Can you work these out from the model? Positions are in its coordinate system, mm. A direction names the side the tool comes from. Round coordinates to 2 decimals unless told otherwise and drop trailing zeros. Loops run counter-clockwise (first coordinate to the right, second up) from the corner with the lowest first, then second, coordinate; pieces in that order, holes last. Notation, with made-up numbers: (44.25, -29.5) -> (95.25, -29.5) arc R33 ccw to (95.25, 6.5) -> close; hole circle Ø3 at (74, 41). An arc over 180 degrees is marked (long way). Answer as a JSON object with one key per item and string values.
```python
from build123d import *

# Parameters (mm, degrees)
F0_W      = 114.3
F0_H      = 69.85
F1_DEPTH  = 50.8
F3_DEPTH  = 76.2
F4_DEPTH  = 19.05
F6_DEPTH  = 12.7
F8_DEPTH  = 76.2
F10_DEPTH = 38.1
F12_DEPTH = 76.2
F14_DEPTH = 12.7
F15_R     = 3.175
F16_DEPTH = 76.2


with BuildPart() as f1:
    # F0 (on Front) → F1 (new body)
    with BuildSketch(Plane.XZ):
        with Locations((57.15, 34.925)):
            Rectangle(F0_W, F0_H)
    extrude(amount=-F1_DEPTH)

    # F2 (on face) → F3 (cut)
    with BuildSketch(Plane.XZ):
        Polygon((0, 0), (63.5, 0), (0, 31.75), align=None)
    extrude(amount=-F3_DEPTH, mode=Mode.SUBTRACT)

    # F2 (on face) → F4 (cut)
    with BuildSketch(Plane.XZ):
        Polygon((38.1, 69.85), (114.3, 50.8), (114.3, 69.85), align=None)
    extrude(amount=-F4_DEPTH, mode=Mode.SUBTRACT)

    # F5 (on face) → F6 (cut)
    with BuildSketch(Plane(origin=(0, 50.8, 0), x_dir=(-1, 0, 0), z_dir=(0, 1, 0))):
        Polygon((-114.3, 50.8), (-38.1, 69.85), (-114.3, 69.85), align=None)
    extrude(amount=-F6_DEPTH, mode=Mode.SUBTRACT)

    # F7 (on face) → F8 (cut)
    with BuildSketch(Plane.XZ.offset(-19.05)):
        Polygon((101.6, 53.975), (101.6, 69.85), (38.1, 69.85), align=None)
    extrude(amount=-F8_DEPTH, mode=Mode.SUBTRACT)

    # F9 (on face) → F10 (join)
    with BuildSketch(Plane.YZ.offset(114.3)):
        Polygon((38.1, 69.85), (19.05, 69.85), (19.05, 50.8), (19.05, 0), (50.8, 0), (50.8, 50.8), (38.1, 50.8), align=None)
    extrude(amount=F10_DEPTH)

    # F11 (on face) → F12 (cut)
    with BuildSketch(Plane.XZ.offset(-19.05)):
        Polygon((139.7, 69.85), (139.7, 31.75), (152.4, 25.4), (152.4, 69.85), align=None)
    extrude(amount=-F12_DEPTH, mode=Mode.SUBTRACT)

    # F13 (on face) → F14 (cut)
    with BuildSketch(Plane(origin=(0, 50.8, 0), x_dir=(-1, 0, 0), z_dir=(0, 1, 0))):
        Polygon((-139.7, 31.75), (-114.3, 50.8), (-139.7, 50.8), align=None)
    extrude(amount=-F14_DEPTH, mode=Mode.SUBTRACT)

    # F15 (on face) → F16 (cut)
    with BuildSketch(Plane.XY.offset(69.85)):
        with Locations((111.125, 28.575)):
            Circle(F15_R)
        with Locations((130.175, 28.575)):
            Circle(F15_R)
    extrude(amount=-F16_DEPTH, mode=Mode.SUBTRACT)


solid = f1.part
```
Q1. I'm going to push flat-ended pins straight in: pin 1 (9.5 mm diameter, centred on y = 31, z = 43, fed in from +X); pin 2 (9.5 mm diameter, centred on y = 13, z = 25.5, fed in from +X); pin 3 (1 mm diameter, centred on y = 40, z = 50, fed in from +X). Where does each tip first touch, or does it pass through?
Determined:
{"pin 1": "x = 139.7", "pin 2": "x = 114.3", "pin 3": "x = 116.03"}
Q2. We'd pull the mould along X, two halves only. Please class faces 6 (the flat face through (139.7, 28, 51)), 7 (the flat face through (125, 38.1, 55)), 8 (the cylindrical face through (133.11, 27.36, 35.41)): pulls with the +X half, pulls with the -X half, needs draft (parallel to the pull), parting line crosses it, or undercut.
Determined:
{"face 6": "pulls with the +X half", "face 7": "needs draft", "face 8": "undercut"}
Q3. I want a section at B-B, the plane x = 111. Write out the boundary of the cut face in (y, z) (3 decimals), then the cut area to 3 significant figures.
Determined:
{"outline": "(0, 0) -> (25.402, 0) -> (25.402, 69.85) -> (19.05, 69.85) -> (19.05, 51.625) -> (0, 51.625) -> close; (31.748, 0) -> (50.8, 0) -> (50.8, 51.625) -> (38.1, 51.625) -> (38.1, 69.85) -> (31.748, 69.85) -> close", "area": "2,530 mm²"}
Q4. On a 3-axis mill with a long thin cutter (end or side, diameter ignored), from which of +Z, -Z, +X, -X, +Y, -Y can I reach the whole of each face in a straight line? I mean faces 1 (the flat face through (127.18, 44.54, 41.14)), 2 (the flat face through (152.4, 35, 13)), 3 (the cylindrical face through (114.06, 27.36, 35.41)), 4 (the flat face through (101.6, 28, 62)), 5 (the flat face through (114.3, 9, 25)). Say none if no direction works.
Determined:
{"face 1": "+Z, +X, +Y", "face 2": "+Z, -Z, +X, +Y, -Y", "face 3": "+Z, -Z", "face 4": "+Z, +Y, -Y", "face 5": "+Z, -Z, +X, -Y"}
Q5. If I drill on L1, parallel to X at y = 26.5, z = 41.5; L2, parallel to X at y = 31, z = 45; L3, parallel to Y at x = 134.5, z = 32.5, over which ranges is the centre line in solid material (lowest first)? Write a range as [from, to].
Determined:
{"L1": "[0, 108.72], [113.53, 127.77], [132.58, 139.7]", "L2": "[0, 109.08], [113.17, 128.13], [132.22, 139.7]", "L3": "[19.05, 50.8]"}
Q6. I want a section at D-D, the plane z = 41. Write out the boundary of the cut face in (x, y) (3 decimals), then the cut area to 3 significant figures.
Determined:
{"outline": "(0, 0) -> (114.3, 0) -> (114.3, 19.05) -> (139.7, 19.05) -> (139.7, 38.1) -> (127.367, 38.1) -> (127.367, 50.8) -> (0, 50.8) -> close; hole circle Ø6.35 at (111.125, 28.575); hole circle Ø6.35 at (130.175, 28.575)", "area": "6,390 mm²"}
Q7. I want a section at C-C, the plane y = 5. Write out the boundary of the cut face in (x, z).
Determined:
{"outline": "(0, 31.75) -> (63.5, 0) -> (114.3, 0) -> (114.3, 50.8) -> (38.1, 69.85) -> (0, 69.85) -> close"}
Q8. I want a section at A-A, the plane z = 63.5. Write out the boundary of the cut face in (x, y) (3 decimals).
Determined:
{"outline": "(0, 0) -> (63.5, 0) -> (63.5, 50.8) -> (0, 50.8) -> close; (101.6, 19.05) -> (139.7, 19.05) -> (139.7, 38.1) -> (101.6, 38.1) -> close; hole circle Ø6.35 at (111.125, 28.575); hole circle Ø6.35 at (130.175, 28.575)"}
